Part model, mm, in its own coordinate system. Face numbers are marked on the shaded views. A direction names the side the tool comes from. Round coordinates to 2 decimals unless told otherwise and drop trailing zeros. Loops run counter-clockwise (first coordinate to the right, second up) from the corner with the lowest first, then second, coordinate; pieces in that order, holes last.
from build123d import *

# Parameters (mm, degrees)
ESBO_O1_W                = 30
ESBO_O1_H                = 30
ESBO_O1_R                = 2
RESSALTO_EXTRUS_O1_DEPTH = 5
ESBO_O2_W                = 30
ESBO_O2_H                = 20
ESBO_O2_R                = 2
RESSALTO_EXTRUS_O2_DEPTH = 5


with BuildPart() as part:
    # Esboço1 → Ressalto-extrusão1 (new body)
    with BuildSketch(Plane.XY):
        Rectangle(ESBO_O1_W, ESBO_O1_H)
        with Locations((-9, 9)):
            Circle(ESBO_O1_R, mode=Mode.SUBTRACT)
        with Locations((9, 9)):
            Circle(ESBO_O1_R, mode=Mode.SUBTRACT)
    extrude(amount=RESSALTO_EXTRUS_O1_DEPTH)

    # Esboço2 → Ressalto-extrusão2 (add)
    with BuildSketch(Plane.XZ.offset(15)):
        with Locations((0, -5)):
            Rectangle(ESBO_O2_W, ESBO_O2_H)
        with Locations((-9, -7)):
            Circle(ESBO_O2_R, mode=Mode.SUBTRACT)
        with Locations((9, -7)):
            Circle(ESBO_O2_R, mode=Mode.SUBTRACT)
    extrude(amount=RESSALTO_EXTRUS_O2_DEPTH)


solid = part.part
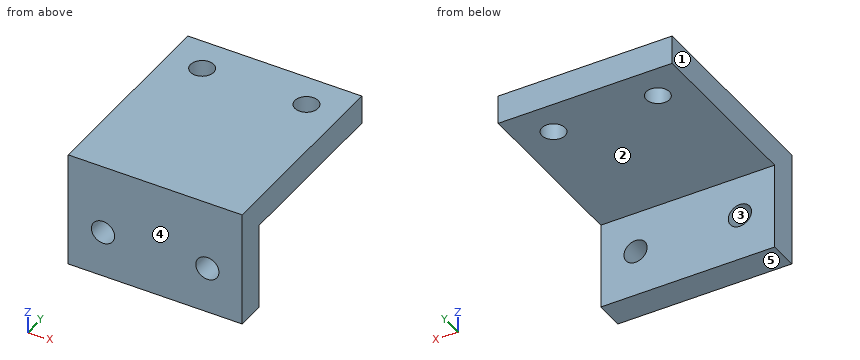
1) Slice it at A-A, the plane z = -7. Give the cut face in (x, y), then the cut area to 3 significant figures.
Values:
outline: (-15, -20) - (-11, -20) - (-11, -15) - (-15, -15) - close; (-7, -20) - (7, -20) - (7, -15) - (-7, -15) - close; (11, -20) - (15, -20) - (15, -15) - (11, -15) - close
area: 110 mm2
2) Slice it at C-C, the plane x = 9. Give the cut face in (y, z).
Values:
outline: (-20, -15) - (-15, -15) - (-15, -9) - (-20, -9) - close; (-20, -5) - (-15, -5) - (-15, 0) - (7, 0) - (7, 5) - (-20, 5) - close; (11, 0) - (15, 0) - (15, 5) - (11, 5) - close
3) Drop flat-ended pins along their axis: pin 1 Ø5 at (x, z) = (9, -7) entering from +Y; pin 2 Ø4 at (y, z) = (0.5, -0.5) entering from +X; pin 3 Ø9 at (x, y) = (2, -6) entering from -Z. Give the stop position or say it passes through.
Values:
pin 1: stops at y = -15
pin 2: stops at x = 15
pin 3: stops at z = 0
4) Slice it at B-B, the plane y = 9. Give the cut face in (x, z), then the cut area to 3 significant figures.
Values:
outline: (-15, 0) - (-11, 0) - (-11, 5) - (-15, 5) - close; (-7, 0) - (7, 0) - (7, 5) - (-7, 5) - close; (11, 0) - (15, 0) - (15, 5) - (11, 5) - close
area: 110 mm2
5) Tool access for the marked faces 1 and 2: list every direction of +Z, -Z, +X, -X, +Y, -Y with a clear straight run to the whole face (end or side of a thin tool).
Values:
face 1: +Z, -Z, -X, +Y, -Y
face 2: -Z, +X, -X, +Y
6) Wall check: line 1 along Y through (x, z) = (-9, 2.5); line 2 along Z through (x, y) = (-9, -17.7); line 3 along Y through (x, z) = (-4.5, -5.25). Give the ranges that are in metal, low to high.
Values:
line 1: y = -20 to 7, 11 to 15
line 2: z = -15 to -9, -5 to 5
line 3: y = -20 to -15
7) Slice it at D-D, the plane z = 2.75. Give the cut face in (x, y), then the cut area to 3 significant figures.
Values:
outline: (-15, -20) - (15, -20) - (15, 15) - (-15, 15) - close; hole circle Ø4 at (-9, 9); hole circle Ø4 at (9, 9)
area: 1,020 mm2
8) Mould opens along Z. For the marked faces 3, 4 and 5 say: released by +Z, released by -Z, zero draft, split by the parting line, or undercut.
Values:
face 3: undercut
face 4: zero draft
face 5: released by -Z
